Verification items for the finished model (mm, model axes). Face numbers are marked on the shaded views. A direction names the side the tool comes from. Coordinates: 2 decimals unless noted, no trailing zeros. Write each loop counter-clockwise with the first axis right and the second up, starting at its lowest first coordinate (ties: lowest second). Pieces come first, ordered by that corner, then holes. Notation, with made-up numbers: M -32.5,10.5 L 16.5,10.5 A23 cw 16.5,23.5 Z; hole C 74,70 d3. An arc over 180 degrees is marked long. Answer in a Markdown table with one row per item.
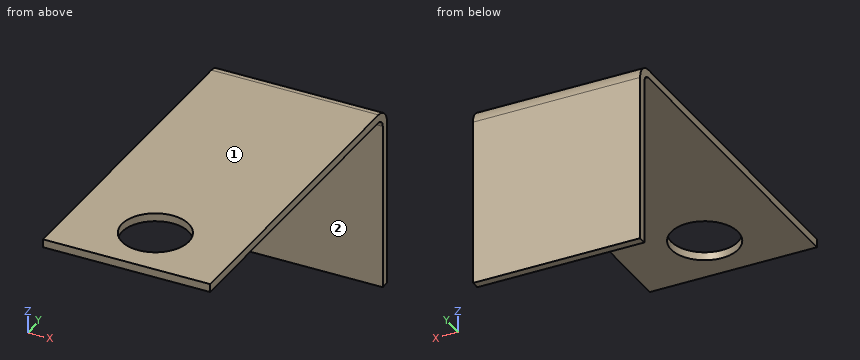
from build123d import *

# Parameters (mm, degrees)
SKETCH1_W               = 15
SKETCH1_H               = 15
BASE_FLANGE1_DEPTH      = 0.7366
EDGE_FLANGE1_DEPTH      = 15
EDGE_FLANGE1_START      = -0.7366
EDGE_FLANGE1_PROFILE_W  = 15
EDGE_FLANGE1_PROFILE_H  = 29.2634
EDGE_FLANGE1_PROFILE_R  = 3
EDGE_FLANGE1_FLAT_DEPTH = 0.7366


# Sheet-metal steps are written as plain solids
with BuildPart() as part:
    # Sketch1 → Base-Flange1 (new body)
    with BuildSketch(Plane(origin=(0, 0, 0), x_dir=(1, 0, 0), z_dir=(0, 1, 0))):
        Rectangle(SKETCH1_W, SKETCH1_H)
    extrude(amount=-BASE_FLANGE1_DEPTH)

    # Edge-Flange1 bend section (across the edge) → Edge-Flange1 (add)
    with BuildSketch(Plane(origin=(7.5, -0.7366, 8.2366), x_dir=(0, 0, -1), z_dir=(-1, 0, 0))):
        with BuildLine():
            Line((-0.7366, 0.7366), (0, 0.7366))
            ThreePointArc((0, 0.7366), (0.215745145, 0.215745145), (0.7366, 0))
            Line((0.7366, 0), (0.7366, -0.7366))
            ThreePointArc((0.7366, -0.7366), (-0.30510971, -0.30510971), (-0.7366, 0.7366))
        make_face()
    extrude(amount=EDGE_FLANGE1_DEPTH)

    # Edge-Flange1 profile (on flange) → Edge-Flange1 flat (add)
    with BuildSketch(Plane(origin=(0, -0.7366, 8.2366), x_dir=(1, 0, 0), z_dir=(0, 0, -1)).offset(EDGE_FLANGE1_START)):
        with Locations((0, 15.3683)):
            Rectangle(EDGE_FLANGE1_PROFILE_W, EDGE_FLANGE1_PROFILE_H)
        with Locations((0, 25)):
            Circle(EDGE_FLANGE1_PROFILE_R, mode=Mode.SUBTRACT)
    extrude(amount=EDGE_FLANGE1_FLAT_DEPTH)


solid = part.part
1) Sectioned sample at D-D (z = -5.5). Record the cut outline in (x, y), then the cut area to 3 significant figures.
Response values:
| item | result |
|---|---|
| outline | M -7.5,-0.74 L 7.5,-0.74 L 7.5,0 L -7.5,0 Z |
| area | 11.0 mm² |
2) Thickness scan on L1, parallel to Y at x = 3, z = 4; L2, parallel to Z at x = 2.75, y = -3; L3, parallel to Y at x = 0, z = 8.8. Record the ranges inside material, lowest first. Write a range as [from, to].
Response values:
| item | result |
|---|---|
| L1 | y = [-0.74, 0] |
| L2 | z = [8.24, 8.97] |
| L3 | y = [-30.74, -28.74], [-22.74, -0.78] |
3) Depth check by flat-ended pin: pin 1 (1.5 mm diameter, centred on x = 4, z = -1.5, fed in from -Y); pin 2 (6 mm diameter, centred on y = -17.5, z = 7, fed in from -X); pin 3 (5 mm diameter, centred on x = 0, y = -25, fed in from -Z). Enter the tip coordinate at first touch or a pass-through.
Response values:
| item | result |
|---|---|
| pin 1 | stops at y = -0.74 |
| pin 2 | stops at x = -7.5 |
| pin 3 | stops at z = 8.24 |
4) Sectioned sample at B-B (x = -6). Record the cut outline in (y, z).
Response values:
| item | result |
|---|---|
| outline | M -30.74,8.24 L -1.47,8.24 A0.74 cw -0.74,7.5 L -0.74,-7.5 L 0,-7.5 L 0,7.5 A1.47 ccw -1.47,8.97 L -30.74,8.97 Z |
5) Tool access check on the marked faces 1 and 2. Record the directions out of +Z, -Z, +X, -X, +Y, -Y that give a thin tool (end or side, any length) a straight path to the whole face; none if there is none.
Response values:
| item | result |
|---|---|
| face 1 | +Z, +X, -X, +Y, -Y |
| face 2 | -Z, +X, -X, -Y |
6) Sectioned sample at A-A (x = 0). Record the cut outline in (y, z).
Response values:
| item | result |
|---|---|
| outline | M -30.74,8.24 L -28.74,8.24 L -28.74,8.97 L -30.74,8.97 Z; M -22.74,8.24 L -1.47,8.24 A0.74 cw -0.74,7.5 L -0.74,-7.5 L 0,-7.5 L 0,7.5 A1.47 ccw -1.47,8.97 L -22.74,8.97 Z |
7) Sectioned sample at C-C (y = -26.5). Record the cut outline in (x, z), then the cut area to 3 significant figures.
Response values:
| item | result |
|---|---|
| outline | M -7.5,8.24 L -2.9,8.24 L -2.9,8.97 L -7.5,8.97 Z; M 2.9,8.24 L 7.5,8.24 L 7.5,8.97 L 2.9,8.97 Z |
| area | 6.77 mm² |
